Verification items for the finished model (mm, model axes). Face numbers are marked on the shaded views. A direction names the side the tool comes from. Coordinates: 2 decimals unless noted, no trailing zeros. Write each loop counter-clockwise with the first axis right and the second up, starting at its lowest first coordinate (ties: lowest second). Pieces come first, ordered by that corner, then holes. Notation, with made-up numbers: (87, 21.5) -> (100, 21.5) arc R25 cw to (100, 59.5) -> close; hole circle Ø4 at (3.25, -26). An arc over 180 degrees is marked (long way). Answer in a Markdown table with one row per item.
```python
from build123d import *

# Parameters (mm, degrees)
F0_R      = 95
F1_DEPTH  = 400
F2_R      = 100
F2_R_2    = 95
F3_DEPTH  = 20
F4_W      = 20
F4_H      = 20
F5_DEPTH  = 5
F6_W      = 60
F6_H      = 60
F6_W_2    = 20
F6_H_2    = 20
F7_W      = 20
F7_H      = 20
F8_DEPTH  = 60
F10_DEPTH = 130.001
F11_R     = 20
F12_DEPTH = 25
F13_W     = 15
F13_H     = 15
F14_DEPTH = 5
F15_R     = 20
F15_W     = 15
F15_H     = 15
F16_DEPTH = 25


with BuildPart() as f1:
    # F0 (on Top) → F1 (new body)
    with BuildSketch(Plane.XY):
        Circle(F0_R)
    extrude(amount=F1_DEPTH)

    # F2 (on face) → F3 (join)
    with BuildSketch(Plane.XY.offset(400)):
        Circle(F2_R)
        Circle(F2_R_2, mode=Mode.SUBTRACT)
        Circle(F2_R_2)
    extrude(amount=F3_DEPTH)

    # F4 (on face) → F5 (join)
    with BuildSketch(Plane.XY.offset(420)):
        Rectangle(F4_W, F4_H)
    extrude(amount=F5_DEPTH)

    # F6 (on face) + F7 (on face) → F8 (join)
    with BuildSketch(Plane.XY.offset(425)):
        Rectangle(F6_W, F6_H)
        Rectangle(F6_W_2, F6_H_2, mode=Mode.SUBTRACT)
    with BuildSketch(Plane.XY.offset(425)):
        Rectangle(F7_W, F7_H)
    extrude(amount=F8_DEPTH)

    # F9 (on face) → F10 (cut, through all)
    with BuildSketch(Plane.XZ.offset(30)):
        Polygon((-27.5, 427.5), (0, 427.5), (27.5, 427.5), (27.5, 482.5), (0, 482.5), (-27.5, 482.5), align=None)
    extrude(amount=-F10_DEPTH, mode=Mode.SUBTRACT)

    # F11 (on face) → F12 (cut)
    with BuildSketch(Plane.XY.offset(485)):
        Circle(F11_R)
    extrude(amount=-F12_DEPTH, mode=Mode.SUBTRACT)

    # F13 (on face) → F14 (join)
    with BuildSketch(Plane.XY.offset(427.5)):
        Rectangle(F13_W, F13_H)
    extrude(amount=F14_DEPTH)

    # F15 (on face) → F16 (join)
    with BuildSketch(Plane.XY.offset(432.5)):
        Circle(F15_R)
        Rectangle(F15_W, F15_H, mode=Mode.SUBTRACT)
        Rectangle(F15_W, F15_H)
    extrude(amount=F16_DEPTH)


solid = f1.part
```
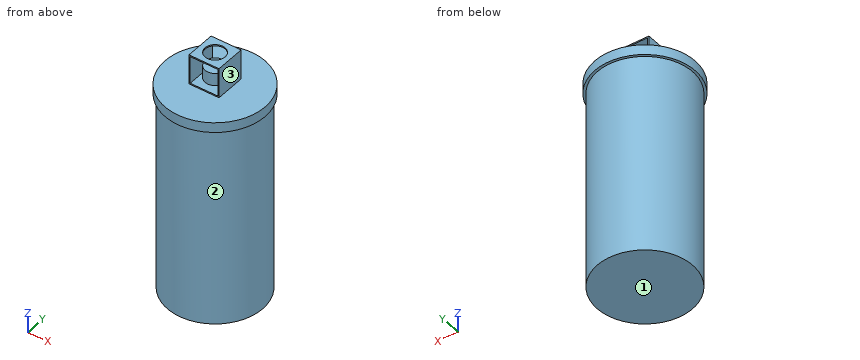
1. Sectioned sample at D-D, the plane x = 59. Record the cut outline in (y, z).
Findings below:
| item | result |
|---|---|
| outline | (-80.74, 400) -> (-74.46, 400) -> (-74.46, 0) -> (74.46, 0) -> (74.46, 400) -> (80.74, 400) -> (80.74, 420) -> (-80.74, 420) -> close |
2. Material ranges on probe 1 along Z at (x, y) = (-23, -22); probe 2 along Y at (x, z) = (0, 483); probe 3 along Z at (x, y) = (29, 0), recorded low to high. Write a range as from..to.
Findings below:
| item | result |
|---|---|
| probe 1 | z = 0..420, 425..427.5, 482.5..485 |
| probe 2 | y = -30..-20, 20..30 |
| probe 3 | z = 0..420, 425..485 |
3. Access from +Z, -Z, +X, -X, +Y, -Y to the whole of each face (thin tool, end or side, straight path). Record for the marked faces 1, 2 and 3.
Findings below:
| item | result |
|---|---|
| face 1 | -Z, +X, -X, +Y, -Y |
| face 2 | -Z |
| face 3 | +Z, +X, +Y, -Y |
4. Go/stop test with flat-tipped pins: pin 1 (8 mm diameter, centred on y = -27.5, z = 169, fed in from +X); pin 2 (12 mm diameter, centred on y = 1, z = 299, fed in from -X); pin 3 (1.5 mm diameter, centred on x = 54, y = -28.5, fed in from -Z); pin 4 (2.5 mm diameter, centred on x = -1, z = 429.5, fed in from +Y). Record where each tip stops, or that it passes through.
Findings below:
| item | result |
|---|---|
| pin 1 | stops at x = 92.05 |
| pin 2 | stops at x = -95 |
| pin 3 | stops at z = 0 |
| pin 4 | stops at y = 7.5 |
5. Sectioned sample at C-C, the plane z = 408. Record the cut outline in (x, y), and give its area (3 significant figures).
Findings below:
| item | result |
|---|---|
| outline | circle Ø200 at (0, 0) |
| area | 31,400 mm² |
6. Sectioned sample at A-A, the plane x = 0. Count the separate pieces of the cut face and the enclosed holes in it, and give its area (3 significant figures).
Findings below:
| item | result |
|---|---|
| separate pieces | 3 |
| enclosed holes | 0 |
| area | 81,400 mm² |
